Could you check a few things on this model? Use its own coordinates, in mm. A direction names the side the tool comes from. Give positions to 0.01 mm unless a question says otherwise; leave off trailing zeros. Order: outer loops, then holes, each group sorted by start corner. A loop starts at its lowest first (then second) coordinate and runs counter-clockwise, first axis right, second up.
(1) Imagine slicing it at A-A, the plane x = 25.25. Write out the boundary of the cut face in (y, z) (3 decimals), then the cut area to 3 significant figures.
(2) Imagine slicing it at B-B, the plane y = 1.45. Write out the boundary of the cut face in (x, z) (3 decimals), then the cut area to 3 significant figures.
(3) If we mould it in two halves opening along X, with no side actions, what happens to faces 1 (the flat face through (17, 2, -35.25)), 2 (the cylindrical face through (21.912, 1.972, -60.926)), 3 (the flat face through (15.25, 2, -6))? For each: released by +X, released by -X, zero draft, split by the parting line, or undercut.
(4) On a 3-axis mill with a long thin cutter (end or side, diameter ignored), from which of +Z, -Z, +X, -X, +Y, -Y can I reach the whole of each face in a straight line? I mean faces 4 (the flat face through (19, 2, -47)), 5 (the flat face through (25, 0, -23)). Say none if no direction works.
(5) Imagine slicing it at C-C, the plane z = -42. Write out the boundary of the cut face in (x, y).
(6) If I drill on probe 1 along Z at (x, y) = (25.25, 3) (3 decimals); probe 2 along Z at (x, y) = (27.5, 1.65) (3 decimals); probe 3 along X at (y, z) = (3.65, -56), over which ranges is the centre line in solid material (lowest first)?
Autodesk Inventor part; units mm, degrees
ref_plane "YZ Plane" through (0, 0, 0) normal (1, 0, 0) x (0, 1, 0)
ref_plane "XZ Plane" through (0, 0, 0) normal (0, 1, 0) x (-1, 0, 0)
ref_plane "XY Plane" through (0, 0, 0) normal (0, 0, 1) x (1, 0, 0)
sketch "Sketch1" plane through (0, 0, 0) normal (0, 1, 0) x (-1, 0, 0)
  circle A0 centre (0, 0) radius 10.5
  line L0 (0, 0) -> (0, -23.5)
  circle A1 centre (0, -23.5) radius 5.25
  line L1 (0, -23.5) -> (0, -35.25)
  line L2 (-14, -35.25) -> (-14, -58.75)
  line L3 (-14, -58.75) -> (-19, -58.75)
  line L4 (-19, -58.75) -> (-19, -35.25)
  line L5 (-35.25, 21.625) -> (35.25, 21.625) construction
  line L6 (35.25, 21.625) -> (25.25, 21.625)
  line L7 (-35.25, -69.875) -> (-35.25, 21.625)
  line L8 (-35.25, 21.625) -> (-35.25, 11.625)
  line L9 (-35.25, 11.625) -> (-25.25, 11.625)
  circle A2 centre (-25.25, 11.625) radius 3.5
  line L10 (35.25, 21.625) -> (25.25, 21.625)
  line L11 (25.25, 21.625) -> (25.25, 11.625)
  circle A3 centre (25.25, 11.625) radius 3.5
  line L12 (35.25, -69.875) -> (25.25, -69.875)
  line L13 (25.25, -69.875) -> (25.25, -59.875)
  circle A4 centre (25.25, -59.875) radius 3.5
  line L14 (-35.25, -69.875) -> (-25.25, -69.875)
  line L15 (-25.25, -69.875) -> (-25.25, -59.875)
  circle A5 centre (-25.25, -59.875) radius 3.5
  line L16 (-25.25, 11.625) -> (-25.25, -18.375)
  circle A6 centre (-25.25, -18.375) radius 2.5
  circle A7 centre (25.25, -29.875) radius 2.5
  line L17 (-19, -35.25) -> (-14, -35.25)
  line L18 (-35.25, 21.625) -> (-15.25, 21.625)
  line L19 (35.25, 21.625) -> (35.25, 11.625)
  line L20 (35.25, -58.75) -> (35.25, -69.875)
  line L21 (35.25, -69.875) -> (25.25, -69.875)
  line L22 (-15.25, -69.875) -> (-35.25, -69.875)
  line L23 (-35.25, 21.625) -> (-15.25, 21.625)
  line L24 (25.25, 21.625) -> (35.25, 21.625)
  line L25 (-35.25, 21.625) -> (-15.25, 21.625)
  line L26 (25.25, 21.625) -> (35.25, 21.625)
  line L27 (25.25, -59.875) -> (25.25, -56.375)
  line L28 (25.25, -32.375) -> (25.25, -29.875)
  line L29 (-15.25, 21.625) -> (-15.25, -35.25)
  line L30 (-15.25, -58.75) -> (-15.25, -69.875)
  dimension "d53" = 7
  dimension "d63" = 5
  dimension "d0" = 21
  dimension "d1" = 23.5
  dimension "d2" = 10.5
  dimension "d3" = 11.75
  dimension "d5" = 23.5
  dimension "d6" = 5
  dimension "d7" = 23.5
  dimension "d9" = 70.5
  dimension "d41" = 70.5
  dimension "d42" = 91.5
  dimension "d43" = 10
  dimension "d44" = 10
  dimension "d45" = 7
  dimension "d46" = 10
  dimension "d47" = 10
  dimension "d48" = 90
  dimension "d50" = 7
  dimension "d51" = 10
  dimension "d52" = 10
  dimension "d54" = 10
  dimension "d55" = 10
  dimension "d56" = 7
  dimension "d60" = 30
  dimension "d61" = 30
  dimension "d62" = 5
  dimension "d65" = 20
extrude "Extrusion1" add sketch "Sketch1" along normal blind 4 contours L17 L4 L3 L30 L22 L14 L7 L18 L29
properties part number "m"
Answer block:
1. outline: (0, -69.875) - (4, -69.875) - (4, -63.375) - (0, -63.375) - close; (0, -56.375) - (4, -56.375) - (4, -20.875) - (0, -20.875) - close; (0, -15.875) - (4, -15.875) - (4, 8.125) - (0, 8.125) - close; (0, 15.125) - (4, 15.125) - (4, 21.625) - (0, 21.625) - close
1. area: 290 mm2
2. outline: (15.25, -69.875) - (35.25, -69.875) - (35.25, 21.625) - (15.25, 21.625) - (15.25, -35.25) - (19, -35.25) - (19, -58.75) - (15.25, -58.75) - close; hole circle Ø7 at (25.25, -59.875); hole circle Ø7 at (25.25, 11.625); hole circle Ø5 at (25.25, -18.375)
2. area: 1,650 mm2
3. face 1: zero draft
3. face 2: undercut
3. face 3: released by -X
4. face 4: -X, +Y, -Y
4. face 5: +Z, -Z, +X, -X, -Y
5. outline: (19, 0) - (35.25, 0) - (35.25, 4) - (19, 4) - close
6. probe 1: z = -69.875 to -63.375, -56.375 to -20.875, -15.875 to 8.125, 15.125 to 21.625
6. probe 2: z = -69.875 to -62.556, -57.194 to -19.465, -17.285 to 8.944, 14.306 to 21.625
6. probe 3: x = 19 to 35.25
